Autodesk Inventor part; units mm, degrees
ref_plane "YZ Plane" through (0, 0, 0) normal (1, 0, 0) x (0, 1, 0)
ref_plane "XZ Plane" through (0, 0, 0) normal (0, 1, 0) x (-1, 0, 0)
ref_plane "XY Plane" through (0, 0, 0) normal (0, 0, 1) x (1, 0, 0)
sketch "Sketch1" plane through (0, 0, 0) normal (0, 1, 0) x (-1, 0, 0)
  line L0 (0, 0) -> (50.927, 0)
  line L1 (50.927, 0) -> (50.927, 38.1)
  line L2 (50.927, 38.1) -> (0, 38.1)
  line L3 (0, 38.1) -> (0, 0)
  dimension "d0" = 50.927
  dimension "d1" = 38.1
extrude "Extrusion1" add sketch "Sketch1" along normal blind 19.05
sketch "Sketch2" plane through (0, 19.05, 0) normal (0, 1, 0) x (1, 0, 0)
  circle A0 centre (-31.877, -19.05) radius 15
  line L0 (-50.927, -38.1) -> (0, -38.1)
  point P0 (-50.927, 0)
  dimension "d4" = 30
  dimension "d5" = 19.05
  dimension "d6" = 19.05
  dimension "d15" = 19.05
extrude "Extrusion2" cut sketch "Sketch2" against normal blind 14
sketch "Sketch3" plane through (-31.877, 5.05, 19.05) normal (0, 1, 0) x (1, 0, 0)
  circle A0 centre (0, 0) radius 15
  circle A1 centre (0, 0) radius 3.175
  circle A2 centre (0, 0) radius 9.0875
  point P0 (31.877, 19.05)
  dimension "d9" = 6.35
  dimension "d12" = 5.9125
  dimension "d13" = 5.9125
extrude "Extrusion3" cut sketch "Sketch3" against normal through all contours A1 | A2
fillet "Fillet1" radius 15 2 edges at (-50.927, 9.525, 0) (-50.927, 9.525, 38.1)
equation "\"d12\" = d13"
properties part number "acmeBearingBlock"
Input: part model. Units: mm. Frame: model coordinates. A direction names the side the tool comes from. Round coordinates to 2 decimals unless told otherwise and drop trailing zeros. Loops run counter-clockwise (first coordinate to the right, second up) from the corner with the lowest first, then second, coordinate; pieces in that order, holes last. Notation, with made-up numbers: (64.25, 25) -> (84.25, 25) arc R25 cw to (84.25, 42) -> close; hole circle Ø7 at (25, -5). An arc over 180 degrees is marked (long way). Use one line per item in the form item = value. Start each with the question number.
Item 1: Material intervals for L1, parallel to X at y = 15, z = 19.05; L2, parallel to X at y = 3.3, z = 19.05; L3, parallel to Z at x = -45.5, y = 12.5, sorted ascending. Write a range as from..to.
Item 2: Set-up query: faces 5 (the face through (-18, 9, 0)), 6 (the face through (-25, 5.05, 26)). Return all of +Z, -Z, +X, -X, +Y, -Y with unobstructed straight access to the full face (end or side cutting, diameter ignored); none if empty.
Item 3: Mould query, pull axis Z, two halves, no side actions, for faces 1 (the face through (-50.927, 9, 19)), 2 (the face through (-46.65, 9.66, 33.59)), 3 (the face through (-46.862, 12.148, 18.39)), 4 (the face through (-46.42, 9.66, 4.28)). Classes: pulls with the +Z half, pulls with the -Z half, needs draft (parallel to the pull), parting line crosses it, or undercut.
Item 4: Section query A-A on z = 19.05. Return the cut outline in (x, y), then the cut area to 3 significant figures.
Item 5: Section query C-C on y = 14.5. Return the cut outline in (x, z).
Item 6: Contact query for flat-ended pins moving along their axis: pin 1 Ø1.5 at (x, z) = (-39.5, 26.5) entering from +Y; pin 2 Ø16.5 at (x, z) = (-31.877, 19.05) entering from +Y. Output: stop coordinate, or through.
Item 7: Section query D-D on z = 31. Return the cut outline in (x, y), then the cut area to 3 significant figures.
Item 8: Section query B-B on x = -28. Return the cut outline in (y, z), then the cut area to 3 significant figures.
Ans:
q1.L1 = -50.93..-46.88, -16.88..0
q1.L2 = -50.93..-40.96, -22.79..0
q1.L3 = 3.45..12.77, 25.33..34.65
q2.face_5 = -Z, +X, -X, +Y, -Y
q2.face_6 = +Y
q3.face_1 = needs draft
q3.face_2 = pulls with the +Z half
q3.face_3 = undercut
q3.face_4 = pulls with the -Z half
q4.outline = (-50.93, 0) -> (-40.96, 0) -> (-40.96, 5.05) -> (-46.88, 5.05) -> (-46.88, 19.05) -> (-50.93, 19.05) -> close; (-22.79, 0) -> (0, 0) -> (0, 19.05) -> (-16.88, 19.05) -> (-16.88, 5.05) -> (-22.79, 5.05) -> close
q4.area = 458 mm^2
q5.outline = (-50.93, 15) arc R15 ccw to (-35.93, 0) -> (0, 0) -> (0, 38.1) -> (-35.93, 38.1) arc R15 ccw to (-50.93, 23.1) -> close; hole circle Ø30 at (-31.88, 19.05)
q6.pin_1 = 5.05
q6.pin_2 = through
q7.outline = (-48.68, 0) -> (0, 0) -> (0, 19.05) -> (-22.81, 19.05) -> (-22.81, 5.05) -> (-40.94, 5.05) -> (-40.94, 19.05) -> (-48.68, 19.05) -> close
q7.area = 673 mm^2
q8.outline = (0, 0) -> (19.05, 0) -> (19.05, 4.56) -> (5.05, 4.56) -> (5.05, 10.83) -> (0, 10.83) -> close; (0, 27.27) -> (5.05, 27.27) -> (5.05, 33.54) -> (19.05, 33.54) -> (19.05, 38.1) -> (0, 38.1) -> close
q8.area = 237 mm^2
